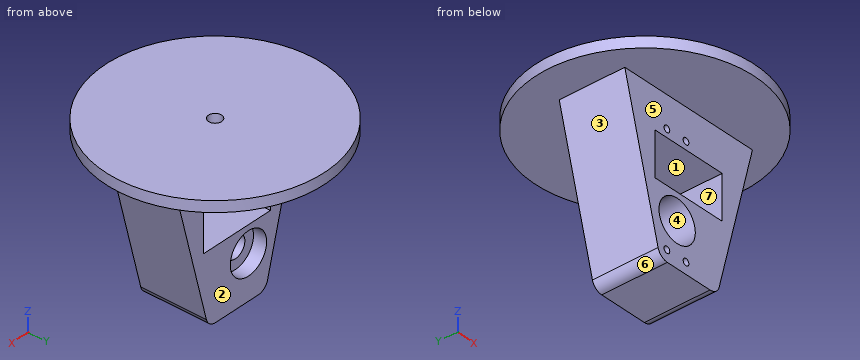
from build123d import *

# Parameters (mm, degrees)
BOSS_EXTRUDE1_DEPTH = 40
SKETCH9_R           = 9.5
CUT_EXTRUDE5_DEPTH  = 20
SKETCH10_R          = 5
CUT_EXTRUDE6_DEPTH  = 21
SKETCH11_R          = 9.5
CUT_EXTRUDE7_DEPTH  = 16
SKETCH14_W          = 35
SKETCH14_H          = 20
CUT_EXTRUDE9_DEPTH  = 41
SKETCH15_R          = 3
CUT_EXTRUDE10_DEPTH = 25
SKETCH16_R          = 50
SKETCH16_R_2        = 3
BOSS_EXTRUDE3_DEPTH = 5
SKETCH17_W          = 69.206254994
SKETCH17_H          = 74.867048483
CUT_EXTRUDE11_DEPTH = 10
SKETCH18_R          = 1.5
CUT_EXTRUDE12_DEPTH = 10
SKETCH20_R          = 1.5
CUT_EXTRUDE13_DEPTH = 10


with BuildPart() as part:
    # Sketch1 → Boss-Extrude1 (new body)
    with BuildSketch(Plane(origin=(0, 0, 0), x_dir=(1, 0, 0), z_dir=(0, 1, 0))):
        with BuildLine():
            Line((-11.141347684, 70), (11.141347684, 70))
            ThreePointArc((11.141347684, 70), (14.196114062, 68.958333283), (15.978061054, 66.267360951))
            Line((15.978061054, 66.267360951), (33.342055813, 0))
            Line((33.342055813, 0), (-33.342055813, 0))
            Line((-33.342055813, 0), (-15.978061054, 66.267360951))
            ThreePointArc((-15.978061054, 66.267360951), (-14.196114062, 68.958333283), (-11.141347684, 70))
        make_face()
    extrude(amount=BOSS_EXTRUDE1_DEPTH)

    # Sketch9 → Cut-Extrude5 (cut)
    with BuildSketch(Plane.XZ):
        with Locations((-6, -50)):
            Circle(SKETCH9_R)
    extrude(amount=-CUT_EXTRUDE5_DEPTH, mode=Mode.SUBTRACT)

    # Sketch10 → Cut-Extrude6 (cut, through all)
    with BuildSketch(Plane.XZ.offset(-20)):
        with Locations((-6, -50)):
            Circle(SKETCH10_R)
    extrude(amount=-CUT_EXTRUDE6_DEPTH, mode=Mode.SUBTRACT)

    # Sketch11 → Cut-Extrude7 (cut)
    with BuildSketch(Plane(origin=(0, 40, 0), x_dir=(1, 0, 0), z_dir=(0, 1, 0))):
        with Locations((-6, 50)):
            Circle(SKETCH11_R)
    extrude(amount=-CUT_EXTRUDE7_DEPTH, mode=Mode.SUBTRACT)

    # Sketch14 → Cut-Extrude9 (cut, through all)
    with BuildSketch(Plane(origin=(0, 40, 0), x_dir=(1, 0, 0), z_dir=(0, 1, 0))):
        with Locations((0, 28)):
            Rectangle(SKETCH14_W, SKETCH14_H)
    extrude(amount=-CUT_EXTRUDE9_DEPTH, mode=Mode.SUBTRACT)

    # Sketch15 → Cut-Extrude10 (cut)
    with BuildSketch(Plane.XY):
        with Locations((0, 20)):
            Circle(SKETCH15_R)
    extrude(amount=-CUT_EXTRUDE10_DEPTH, mode=Mode.SUBTRACT)

    # Sketch16 → Boss-Extrude3 (add)
    with BuildSketch(Plane.XY):
        with Locations((0, 20)):
            Circle(SKETCH16_R)
        with Locations((0, 20)):
            Circle(SKETCH16_R_2, mode=Mode.SUBTRACT)
    extrude(amount=BOSS_EXTRUDE3_DEPTH)

    # Sketch17 → Cut-Extrude11 (cut)
    with BuildSketch(Plane(origin=(0, 40, 0), x_dir=(1, 0, 0), z_dir=(0, 1, 0))):
        with Locations((1.261071684, 37.433524242)):
            Rectangle(SKETCH17_W, SKETCH17_H)
    extrude(amount=-CUT_EXTRUDE11_DEPTH, mode=Mode.SUBTRACT)

    # Sketch18 → Cut-Extrude12 (cut)
    with BuildSketch(Plane.XZ):
        with Locations((-1.350189987, -64.85)):
            Circle(SKETCH18_R)
        with Locations((-11.350189987, -64.85)):
            Circle(SKETCH18_R)
    extrude(amount=-CUT_EXTRUDE12_DEPTH, mode=Mode.SUBTRACT)

    # Sketch20 → Cut-Extrude13 (cut)
    with BuildSketch(Plane.XZ):
        with Locations((-11.350189987, -14.35)):
            Circle(SKETCH20_R)
        with Locations((-1.350189987, -14.35)):
            Circle(SKETCH20_R)
    extrude(amount=-CUT_EXTRUDE13_DEPTH, mode=Mode.SUBTRACT)


solid = part.part
CAD build for the part. Positions are in the model's coordinates, mm. Face numbers are marked on the shaded views. A direction names the side the tool comes from. Round coordinates to 2 decimals unless told otherwise and drop trailing zeros. Loops run counter-clockwise (first coordinate to the right, second up) from the corner with the lowest first, then second, coordinate; pieces in that order, holes last.
(1) Drop flat-ended pins along their axis: pin 1 (10 mm diameter, centred on y = 8, z = -26.5, fed in from -X); pin 2 (0.9 mm diameter, centred on x = -10.5, z = -14, fed in from -Y); pin 3 (8 mm diameter, centred on x = 33.5, z = -9, fed in from +Y); pin 4 (9 mm diameter, centred on x = -6, z = -50, fed in from +Y). Give the stop position or say it passes through.
(2) Which spindle directions (+Z, -Z, +X, -X, +Y, -Y) get a long thin tool onto all of the face, cutting with end or side? Do the marked faces 4, 5, 6 and 7. Say none if no direction does.
(3) Two-plate mould, pull along Z, no slides. Class the marked faces 1, 2 and 3: +Z half, -Z half, draft (parallel to the pull), parting line (faces both ways), or undercut.
(4) Cut at B-B (z = -20.5). Give the cut face in (x, y), plus the area to 3 significant figures.
(5) Cut at A-A (x = -6). Give the cut face in (y, z), plus the area to 3 significant figures.
(6) Cut at C-C (x = 13). Give the cut face in (y, z), plus the area to 3 significant figures.
(7) Wall check: line 1 along Z through (x, y) = (-6, 21.8); line 2 along Y through (x, z) = (0, 1.1); line 3 along X through (y, z) = (6, -14). Give the ranges that are in metal, low to high.
(8) Cut at D-D (y = 14.5). Give the cut face in (x, z).
Findings below:
1. pin 1: stops at x = -27.71
1. pin 2: stops at y = 10
1. pin 3: stops at y = 30
1. pin 4: passes through
2. face 4: -Y
2. face 5: -Z, +X, -X, -Y
2. face 6: -Z, -X, +Y, -Y
2. face 7: +Y, -Y
3. face 1: undercut
3. face 2: draft
3. face 3: -Z half
4. outline: (-27.97, 0) - (-17.5, 0) - (-17.5, 30) - (-27.97, 30) - close; (17.5, 0) - (27.97, 0) - (27.97, 30) - (17.5, 30) - close
4. area: 628 mm2
5. outline: (-29.64, 0) - (0, 0) - (0, -18) - (30, -18) - (30, 0) - (69.64, 0) - (69.64, 5) - (-29.64, 5) - close; (0, -70) - (30, -70) - (30, -59.5) - (24, -59.5) - (24, -55) - (20, -55) - (20, -59.5) - (0, -59.5) - close; (0, -40.5) - (20, -40.5) - (20, -45) - (24, -45) - (24, -40.5) - (30, -40.5) - (30, -38) - (0, -38) - close
5. area: 1,460 mm2
6. outline: (-28.28, 0) - (0, 0) - (0, -18) - (30, -18) - (30, 0) - (68.28, 0) - (68.28, 5) - (-28.28, 5) - close; (0, -69.64) - (30, -69.64) - (30, -38) - (0, -38) - close
6. area: 1,970 mm2
7. line 1: z = -70 to -55, -45 to -38, -18 to 5
7. line 2: y = -30 to 17, 23 to 70
7. line 3: x = -29.67 to -12.81, -9.89 to -2.81, 0.11 to 29.67
8. outline: (-49.7, 0) - (-33.34, 0) - (-15.98, -66.27) arc R5 ccw to (-11.14, -70) - (11.14, -70) arc R5 ccw to (15.98, -66.27) - (33.34, 0) - (49.7, 0) - (49.7, 5) - (-49.7, 5) - close; hole (-17.5, -38) - (17.5, -38) - (17.5, -18) - (-17.5, -18) - close; hole circle Ø19 at (-6, -50)
